from build123d import *

# Parameters (mm, degrees)
SKETCH_1_R      = 8.05
SKETCH_1_W      = 10
SKETCH_1_H      = 2.8
SKETCH_1_W_2    = 5
EXTRUDE_1_DEPTH = 1.4
FILLET_1_R      = 5


with BuildPart() as part:
    # Эскиз1 → Бобышка-Вытянуть1 (new, symmetric)
    with BuildSketch(Plane.XY):
        Polygon((-15, 12.6), (-17.8, 12.6), (-17.8, 7.6), (-15, 7.6), (-15, -7.6), (-17.8, -7.6), (-17.8, -12.6), (-15, -12.6), (-15, -18), (15, -18), (15, -12.6), (17.8, -12.6), (17.8, -7.6), (15, -7.6), (15, 7.6), (17.8, 7.6), (17.8, 12.6), (15, 12.6), (15, 18), (5, 18), (5, 15.2), (-5, 15.2), (-5, 18), (-15, 18), align=None)
        Circle(SKETCH_1_R, mode=Mode.SUBTRACT)
        with Locations((0, -14)):
            Rectangle(SKETCH_1_W, SKETCH_1_H, mode=Mode.SUBTRACT)
        with Locations((9, 14)):
            Rectangle(SKETCH_1_W_2, SKETCH_1_H, mode=Mode.SUBTRACT)
        with Locations((-9, 14)):
            Rectangle(SKETCH_1_W_2, SKETCH_1_H, mode=Mode.SUBTRACT)
    extrude(amount=EXTRUDE_1_DEPTH, both=True)

    # Скругление1
    fillet_1_edges = [part.edges().sort_by_distance(p)[0] for p in [
        (15, 18, 0),
        (15, -18, 0),
        (-15, -18, 0),
        (-15, 18, 0),
    ]]
    fillet(fillet_1_edges, radius=FILLET_1_R)


solid = part.part
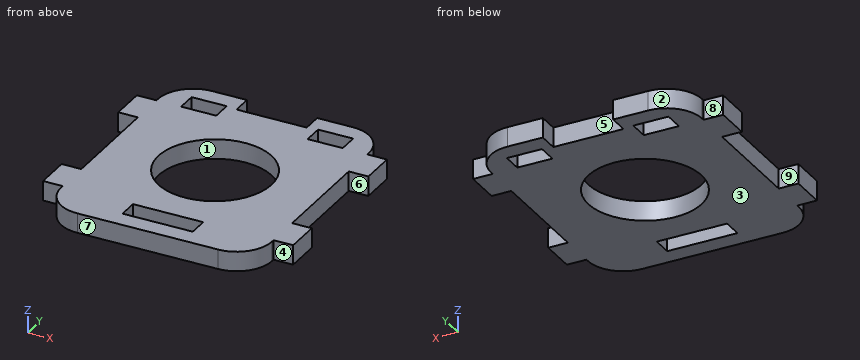
For this review, take the finished solid that the model builds, in its own axes (mm). Face numbers are marked on the shaded views. A direction names the side the tool comes from. Round coordinates to 2 decimals unless told otherwise and drop trailing zeros. Order: outer loops, then holes, each group sorted by start corner. A loop starts at its lowest first (then second) coordinate and runs counter-clockwise, first axis right, second up. Notation, with made-up numbers: (-32, 68) -> (-19, 68) arc R24 cw to (-19, 90) -> close; hole circle Ø10 at (-1.5, 47). An arc over 180 degrees is marked (long way). Put each result on its own line as item: value.
Q1. Insertion check: pin 1 Ø0.8 at (x, z) = (16, -0.5) entering from +Y; pin 2 Ø1.5 at (x, z) = (3, -1) entering from +Y; pin 3 Ø0.8 at (y, z) = (1, 0.5) entering from +X. Each pin has a flat end and moves straight along its axis. Give the tip position at first contact, or say it passes through.
Check result:
pin 1: y = 12.6
pin 2: y = 15.2
pin 3: x = 15
Q2. Machinability: for the marked faces 5, 6, 7, 8 and 9, which of the approach directions +Z, -Z, +X, -X, +Y, -Y give a long, thin tool a straight path to every point of the face, cutting with its end or side? Answer none if there is none.
Check result:
face 5: +Z, -Z, +Y
face 6: +Z, -Z, +X
face 7: +Z, -Z, +X, -X, -Y
face 8: +Z, -Z, -X, +Y
face 9: +Z, -Z, -X
Q3. Add section D-D on z = -0.8. State how many separate pieces and enclosed holes the cut face has, plus the area to 3 significant figures.
Check result:
separate pieces: 1
enclosed holes: 4
area: 827 mm2
Q4. Add section C-C on x = 15.5. Write out the cut boundary in (y, z).
Check result:
outline: (-12.6, -1.4) -> (-7.6, -1.4) -> (-7.6, 1.4) -> (-12.6, 1.4) -> close; (7.6, -1.4) -> (12.6, -1.4) -> (12.6, 1.4) -> (7.6, 1.4) -> close
Q5. Add section B-B on y = 0. Write out the cut boundary in (x, z), plus the area to 3 significant figures.
Check result:
outline: (-15, -1.4) -> (-8.05, -1.4) -> (-8.05, 1.4) -> (-15, 1.4) -> close; (8.05, -1.4) -> (15, -1.4) -> (15, 1.4) -> (8.05, 1.4) -> close
area: 38.9 mm2
Q6. For probe 1 along Y at (x, z) = (0, -0.1); probe 2 along Y at (x, z) = (-8.5, -0.4); probe 3 along Y at (x, z) = (16.5, 1.1), list the stretches that pass through material, from the lowest coordinate up. Write a range as [from, to].
Check result:
probe 1: [-18, -15.4], [-12.6, -8.05], [8.05, 15.2]
probe 2: [-18, 12.6], [15.4, 18]
probe 3: [-12.6, -7.6], [7.6, 12.6]
Q7. Mouldability with a two-part tool opening along Y and no side actions: class the marked faces 1, 2, 3 and 4 as pulls with the +Y half, pulls with the -Y half, needs draft (parallel to the pull), parting line crosses it, or undercut.
Check result:
face 1: undercut
face 2: pulls with the +Y half
face 3: needs draft
face 4: pulls with the -Y half
Q8. Add section A-A on x = 0. Write out the cut boundary in (y, z).
Check result:
outline: (-18, -1.4) -> (-15.4, -1.4) -> (-15.4, 1.4) -> (-18, 1.4) -> close; (-12.6, -1.4) -> (-8.05, -1.4) -> (-8.05, 1.4) -> (-12.6, 1.4) -> close; (8.05, -1.4) -> (15.2, -1.4) -> (15.2, 1.4) -> (8.05, 1.4) -> close
